```python
from build123d import *

# Parameters (mm, degrees)
SKETCH1_R           = 28
BOSS_EXTRUDE1_DEPTH = 7
SKETCH2_R           = 10
CUT_EXTRUDE1_DEPTH  = 41.211938526
SKETCH3_R           = 1.275
CUT_EXTRUDE2_DEPTH  = 41.211938526
CIRPATTERN1_COUNT   = 2


with BuildPart() as part:
    # Sketch1 → Boss-Extrude1 (new body)
    with BuildSketch(Plane(origin=(0, 0, 0), x_dir=(1, 0, 0), z_dir=(0, 1, 0))):
        with Locations(Location((0, 0, 0), (0, 0, 270))):
            Circle(SKETCH1_R)
    extrude(amount=BOSS_EXTRUDE1_DEPTH)

    # Sketch2 → Cut-Extrude1 (cut, through all)
    with BuildSketch(Plane(origin=(0, 0, 0), x_dir=(1, 0, 0), z_dir=(0, 1, 0))):
        with Locations(Location((0, 0, 0), (0, 0, 270))):
            Circle(SKETCH2_R)
    extrude(amount=CUT_EXTRUDE1_DEPTH, mode=Mode.SUBTRACT)

    # Sketch3 → Cut-Extrude2 (cut, through all)
    with BuildSketch(Plane(origin=(0, 0, 0), x_dir=(1, 0, 0), z_dir=(0, 1, 0))):
        with Locations(Location((23.0124, 0, 0), (0, 0, 270))):
            Circle(SKETCH3_R)
    cut_extrude2 = extrude(amount=CUT_EXTRUDE2_DEPTH, mode=Mode.SUBTRACT)

    # CirPattern1: Cut-Extrude2 ×2 about axis
    cirpattern1_axis = Axis((0, 0, 0), (0, 1, 0))
    for i in range(1, CIRPATTERN1_COUNT):
        add(cut_extrude2.rotate(cirpattern1_axis, i * 360 / CIRPATTERN1_COUNT), mode=Mode.SUBTRACT)


solid = part.part
```
Check sheet for the modelled part. Datum: model origin and axes. Units: mm. Give positions to 0.01 mm unless a question says otherwise; leave off trailing zeros. Write each loop counter-clockwise with the first axis right and the second up, starting at its lowest first coordinate (ties: lowest second). Pieces come first, ordered by that corner, then holes.
Item 1: Gauge pin test, flat ends, axial feed: pin 1 (1 mm diameter, centred on x = -21.5, y = 2, fed in from +Z); pin 2 (2 mm diameter, centred on x = 3.5, y = 2, fed in from +Z); pin 3 (1.5 mm diameter, centred on x = -23.01, z = 0, fed in from +Y). Record the tip position at first contact, or that the pin passes through.
Item 2: Cross-section at D-D (y = 3.75). Enter the section's corners in (x, z) (3 decimals).
Item 3: Scan lines: L1, parallel to X at y = 2.75, z = 0; L2, parallel to Z at x = -6, y = 4.5; L3, parallel to Z at x = -8, y = 5. Record each from-to range of solid material in increasing order.
Item 4: Cross-section at A-A (x = 0). Enter the section's corners in (y, z), and give its area (3 significant figures).
Item 5: Cross-section at C-C (z = 9). Enter the section's corners in (x, y), and give its area (3 significant figures).
Item 6: Cross-section at B-B (z = 0). Enter the section's corners in (x, y).
Item 7: Draft check along Z on faces 1 (the face through (-27.334, 3.451, -6.07)), 2 (the face through (-9.76, 3.45, -2.17)), 3 (the face through (0, 7, 12)). Enter one of: released by +Z, released by -Z, zero draft, split by the parting line, or undercut.
Report:
1. pin 1: stops at z = 18.52
1. pin 2: stops at z = 27.89
1. pin 3: passes through
2. outline: circle Ø56 at (0, 0); hole circle Ø2.55 at (-23.012, 0); hole circle Ø20 at (0, 0); hole circle Ø2.55 at (23.012, 0)
3. L1: x = -28 to -24.29, -21.74 to -10, 10 to 21.74, 24.29 to 28
3. L2: z = -27.35 to -8, 8 to 27.35
3. L3: z = -26.83 to -6, 6 to 26.83
4. outline: (0, -28) - (7, -28) - (7, -10) - (0, -10) - close; (0, 10) - (7, 10) - (7, 28) - (0, 28) - close
4. area: 252 mm2
5. outline: (-26.51, 0) - (-4.36, 0) - (-4.36, 7) - (-26.51, 7) - close; (4.36, 0) - (26.51, 0) - (26.51, 7) - (4.36, 7) - close
5. area: 310 mm2
6. outline: (-28, 0) - (-24.29, 0) - (-24.29, 7) - (-28, 7) - close; (-21.74, 0) - (-10, 0) - (-10, 7) - (-21.74, 7) - close; (10, 0) - (21.74, 0) - (21.74, 7) - (10, 7) - close; (24.29, 0) - (28, 0) - (28, 7) - (24.29, 7) - close
7. face 1: split by the parting line
7. face 2: undercut
7. face 3: zero draft
